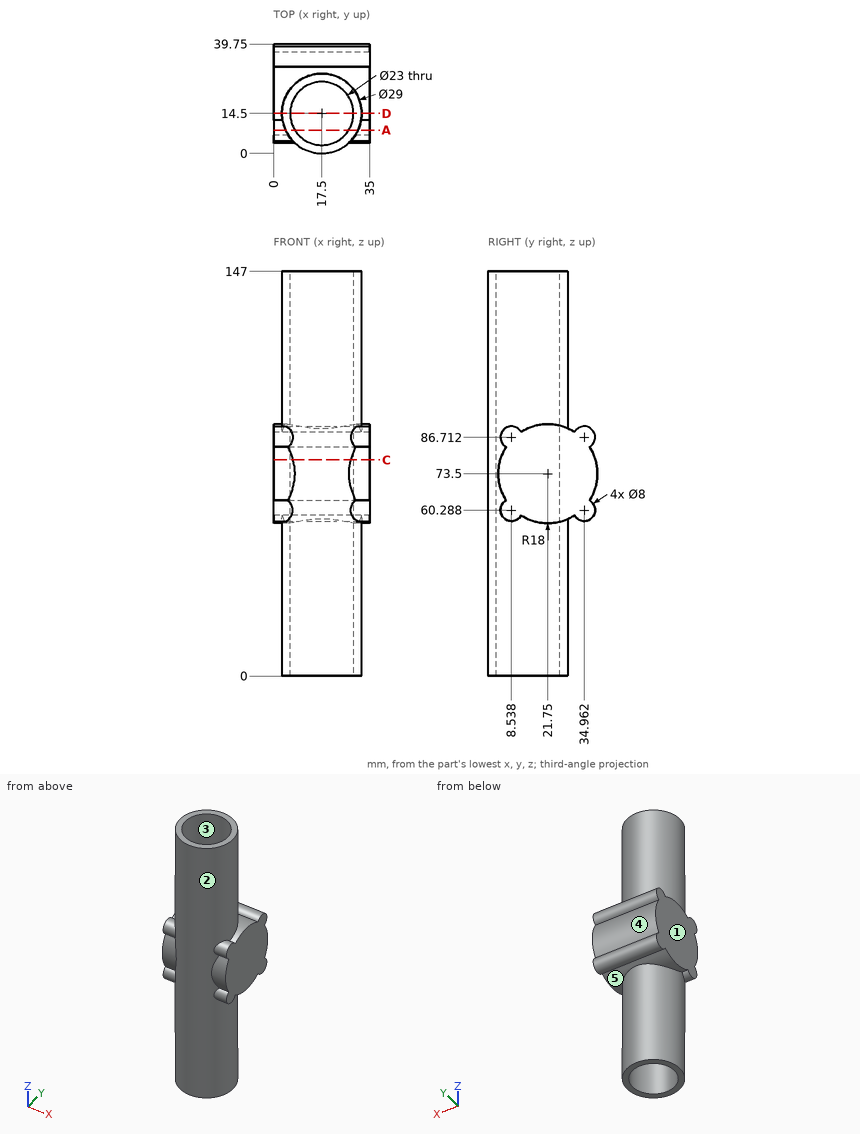
Design review of the part shown in the three views and the two pictorial views. Dimensions are in mm from the part's minimum x, y and z. A direction names the side the tool comes from. Give positions to 0.01 mm unless a question says otherwise; leave off trailing zeros. Loops run counter-clockwise (first coordinate to the right, second up) from the corner with the lowest first, then second, coordinate; pieces in that order, holes last. Notation, with made-up numbers: (41.25, 68) -> (49.25, 68) arc R9 cw to (49.25, 74) -> close; hole circle Ø6 at (25.5, 74). An arc over 180 degrees is marked (long way). Write each question's results on one line, items separated by ' | '.
1) Tool access review of the marked faces 4 and 5: name each direction out of +Z, -Z, +X, -X, +Y, -Y from which nothing blocks a thin tool from reaching the whole face with its end or side.
Conclusion:
face 4: +X, -X, +Y | face 5: -Z
2) Insertion check: pin 1 Ø1 at (x, y) = (21.5, 35) entering from -Z; pin 2 Ø1.5 at (x, z) = (26.5, 108) entering from -Y (1 decimal); pin 3 Ø3 at (x, y) = (13.5, 23) entering from +Z; pin 4 Ø1.5 at (x, z) = (25, 115.5) entering from +Y. Each pin has a flat end and moves straight along its axis. Give the tip position at first contact, or say it passes through.
Conclusion:
pin 1: stops at z = 56.29 | pin 2: stops at y = 2.6 | pin 3: passes through | pin 4: stops at y = 27.33
3) Take a section at A-A, the plane y = 8.5. Give the boundary of the cut face in (x, z), plus the area to 3 significant figures.
Conclusion:
outline: (0, 56.29) -> (4.3, 56.29) -> (4.3, 0) -> (7.69, 0) -> (7.69, 147) -> (4.3, 147) -> (4.3, 90.71) -> (0, 90.71) -> close; (27.31, 0) -> (30.7, 0) -> (30.7, 56.29) -> (35, 56.29) -> (35, 90.71) -> (30.7, 90.71) -> (30.7, 147) -> (27.31, 147) -> close | area: 1,290 mm^2
4) Take a section at C-C, the plane z = 78.5. Give the boundary of the cut face in (x, y).
Conclusion:
outline: (0, 4.46) -> (7.04, 4.46) arc R14.5 ccw to (27.96, 4.46) -> (35, 4.46) -> (35, 39.04) -> (0, 39.04) -> close; hole circle Ø23 at (17.5, 14.5)
5) Draft analysis for pull direction X (two halves, no side actions). For the marked faces 1, 2 and 3, state which applies: pulls with the +X half, pulls with the -X half, needs draft (parallel to the pull), parting line crosses it, or undercut.
Conclusion:
face 1: pulls with the -X half | face 2: parting line crosses it | face 3: undercut
6) For line 1 along X through (y, z) = (14, 97); line 2 along Y through (x, z) = (17, 47); line 3 along Y through (x, z) = (11, 89) (1 decimal), list the stretches that pass through material, from the lowest coordinate up. Write a range as from..to.
Conclusion:
line 1: x = 3.01..6.01, 28.99..31.99 | line 2: y = 0.01..3.01, 25.99..28.99 | line 3: y = 1.5..5, 24..30.9, 31.7..38.2
7) Take a section at D-D, the plane y = 14.5. Give the boundary of the cut face in (x, z) (1 decimal), plus the area to 3 significant figures.
Conclusion:
outline: (0, 57) -> (3, 57) -> (3, 0) -> (6, 0) -> (6, 147) -> (3, 147) -> (3, 90) -> (0, 90) -> close; (29, 0) -> (32, 0) -> (32, 57) -> (35, 57) -> (35, 90) -> (32, 90) -> (32, 147) -> (29, 147) -> close | area: 1,080 mm^2
